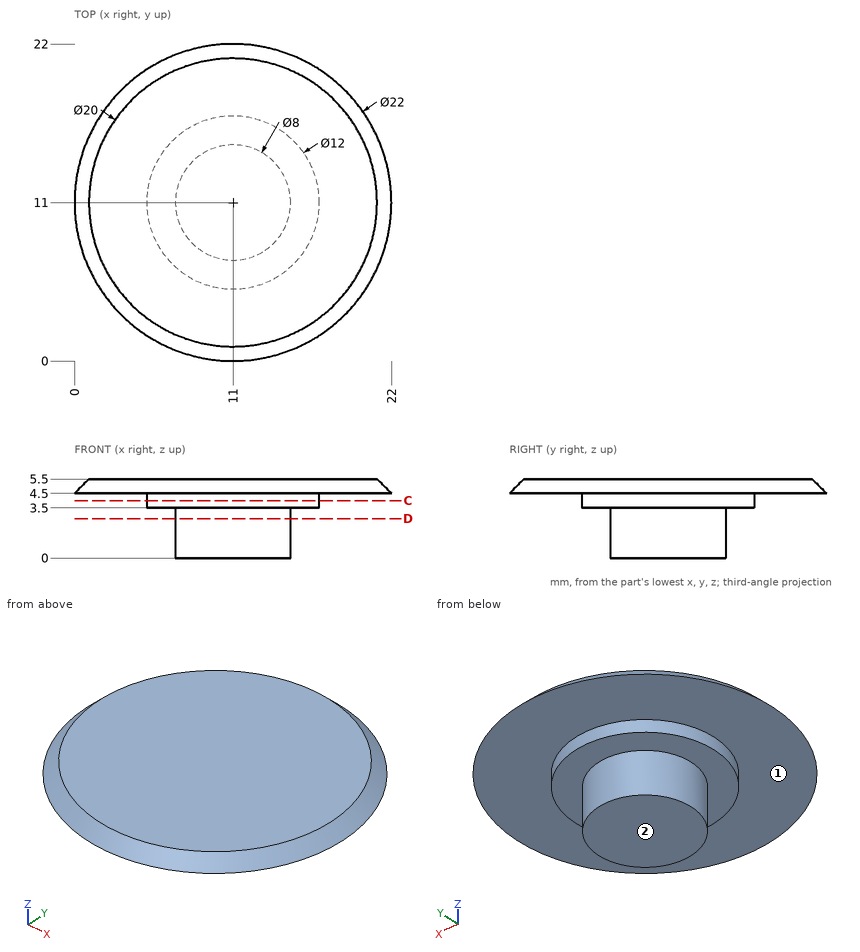
Input: dimensioned drawing with shaded views. Units: mm. Origin: part minimum x, y, z. A direction names the side the tool comes from. Round coordinates to 2 decimals unless told otherwise and drop trailing zeros. Loops run counter-clockwise (first coordinate to the right, second up) from the corner with the lowest first, then second, coordinate; pieces in that order, holes last. Notation, with made-up numbers: (42.5, -27.75) -> (66.5, -27.75) arc R23 ccw to (66.5, 0.25) -> close; hole circle Ø7 at (42.5, 54.25). An arc over 180 degrees is marked (long way). Answer as a JSON object with one key per item and string values. Group by question number.
1) Pin query (flat end, axial travel): pin 1 (6 mm diameter, centred on x = 4, y = 17.5, fed in from -Z). Return the tip coordinate at first contact, or that it passes through.
2) Section query D-D on z = 2.75. Output: boundary loops of the cut face in (x, y).
3) Ray query, L1, parallel to Z at x = 5.75, y = 6.25; L2, parallel to Z at x = 19.75, y = 5.75; L3, parallel to Y at x = 2.5, z = 4.65. Return the intervals inside material, ascending.
4) Section query C-C on z = 4. Output: boundary loops of the cut face in (x, y).
5) Reachability of the marked faces 1 and 2 from +Z, -Z, +X, -X, +Y, -Y: full face, straight path, thin tool, end or side. Return the list, or none.
Reply:
{
 "1": {"pin 1": "stops at z = 4.5"},
 "2": {"outline": "circle Ø8 at (11, 11)"},
 "3": {"L1": "z = 4.5 to 5.5", "L2": "z = 4.5 to 5.3", "L3": "y = 4.26 to 17.74"},
 "4": {"outline": "circle Ø12 at (11, 11)"},
 "5": {"face 1": "-Z", "face 2": "-Z, +X, -X, +Y, -Y"}
}
